The listing builds one solid part. Answer for the finished solid, in the listing's coordinates (mm). Round coordinates to 2 decimals unless told otherwise and drop trailing zeros. Loops run counter-clockwise (first coordinate to the right, second up) from the corner with the lowest first, then second, coordinate; pieces in that order, holes last. Notation, with made-up numbers: (41, 82) - (50, 82) arc R12 ccw to (50, 96) - close; hole circle Ø2 at (-5, -5). An arc over 180 degrees is marked (long way). One line per item, written item: value.
Autodesk Inventor part; units mm, degrees
ref_plane "YZ Plane" through (0, 0, 0) normal (1, 0, 0) x (0, 1, 0)
ref_plane "XZ Plane" through (0, 0, 0) normal (0, 1, 0) x (-1, 0, 0)
ref_plane "XY Plane" through (0, 0, 0) normal (0, 0, 1) x (1, 0, 0)
sketch "Sketch1" plane through (0, 0, 0) normal (0, 0, 1) x (1, 0, 0)
  line L0 (-85.3538, 38.1) -> (162.2962, 38.1)
  line L1 (162.2962, 38.1) -> (162.2962, 12.7)
  line L2 (162.2962, 12.7) -> (-85.3538, 12.7)
  line L3 (-85.3538, 12.7) -> (-85.3538, 38.1)
  line L4 (162.2962, 38.1) -> (115.3062, 38.1)
  line L5 (115.3062, 38.1) -> (115.3062, 0)
  line L6 (115.3062, 0) -> (162.2962, 0)
  line L7 (162.2962, 0) -> (162.2962, 38.1)
  circle A0 centre (-22.5792, -171.9682) radius 173.1686
  line L8 (-85.3538, 12.7) -> (-85.3538, 0)
  line L9 (0, 0) -> (-44.3742, 6.35) construction
  line L10 (-44.3742, 6.35) -> (-85.3538, 0) construction
  spline S0 degree 2 poles (0, 0) (-44.3742, 6.35) (-85.3538, 0) knots 1 1 1 2 2 2
  line L11 (81.5863, -33.6319) -> (69.4058, 12.7)
  line L12 (0, 0) -> (0, 12.7)
  line L13 (0, 0) -> (67.6812, 0)
  line L14 (0, 0) -> (67.6812, 0)
  line L15 (81.5863, -33.6319) -> (29.3756, 0)
  line L16 (0, 0) -> (29.3756, 0)
  line L17 (27.7818, -6.2843) -> (29.3756, 0)
  line L18 (27.7744, -6.2821) -> (21.0977, 0)
  line L19 (7.9763, 0) -> (27.7808, -6.2881)
  line L20 (7.9763, 0) -> (7.5205, -1.4355)
  line L21 (0, 0) -> (7.5205, -1.4355) construction
  spline S1 degree 1 poles (0, 0) (7.5205, -1.4355) knots 1 1 2 2
  line L22 (81.5863, -33.6319) -> (101.3506, -50.0871) construction
  line L23 (101.3506, -50.0871) -> (95.7634, -43.4306) construction
  spline S2 degree 2 poles (81.5863, -33.6319) (101.3506, -50.0871) (95.7634, -43.4306) knots 1 1 1 2 2 2
  line L24 (162.2962, 0) -> (162.2962, -7.7512)
  arc A1 (88.9377, -39.659) -> (162.2962, -7.7512) centre (115.3062, 0) ccw
  arc A2 (162.2962, 7.7512) -> (81.5863, -33.6319) centre (115.3062, 0) ccw
  point P0 (60.3061, -19.9241)
  point P1 (162.2962, 12.7)
  point P2 (115.3062, 12.7)
  point P3 (162.2962, 12.7)
  point P4 (27.497, -6.198)
  point P5 (29.3756, 0)
  point P6 (89.8079, -40.2241)
  dimension "d0" = 247.65
  dimension "d1" = 25.4
  dimension "d4" = 38.1
  dimension "d5" = 46.99
extrude "Extrusion2" add sketch "Sketch1" along normal blind 1.5875 contours L0 A2 L2 L3 | L0 L5 L2 A2 | L2 L12 S0 L8 | L0 A2 L2 L5 | L0 L1 L2 A2 | A2 L13 L12 L2 | L2 L5 L6 L24 A1 A0 L11 | L11 A2 | L2 A2 L7 L6 L5 | L2 L7 A2 | A0 L15 L13 A2 | L13 L20 S1 | A0 L17 L15 | L17 A0 L18 L13 | L13 L18 A0 L19 | L19 A0 L20
fillet "Fillet1" radius 28.575 1 edges at (162.2962, 38.1, 0.7937)
fillet "Fillet2" radius 3.175 1 edges at (-85.3538, 38.1, 0.7937)
fillet "Fillet3" radius 3.175 1 edges at (-85.3538, 0, 0.7937)
sketch "Sketch2" plane through (0, 0, 1.5875) normal (0, 0, 1) x (1, 0, 0)
  circle A0 centre (-77.0322, 20.6187) radius 2.54
  line L0 (-77.0322, 20.6187) -> (-77.0322, 7.9187)
  circle A1 centre (-77.0322, 7.9187) radius 2.54
  line L1 (-77.0322, 20.6187) -> (-13.5322, 20.6187)
  circle A2 centre (-13.5322, 20.6187) radius 2.54
  line L2 (-77.0322, 7.9187) -> (-13.5322, 7.9187)
  circle A3 centre (-13.5322, 7.9187) radius 2.54
  line L3 (-13.5322, 20.6187) -> (-13.5322, 14.2687)
  line L4 (-13.5322, 14.2687) -> (-7.1822, 14.2687)
  circle A4 centre (-7.1822, 14.2687) radius 2.54
  line L5 (-7.1822, 14.2687) -> (5.5178, 14.2687)
  circle A5 centre (5.5178, 14.2687) radius 2.54
  point P0 (0, 0)
  dimension "d15" = 5.08
  dimension "d16" = 12.7
  dimension "d17" = 5.08
  dimension "d18" = 63.5
  dimension "d19" = 5.08
  dimension "d20" = 5.08
  dimension "d21" = 63.5
  dimension "d22" = 6.35
  dimension "d23" = 6.35
  dimension "d24" = 5.08
  dimension "d25" = 12.7
  dimension "d26" = 5.08
properties part number "meers goofy intake sled"
1) Consider L1, parallel to Y at x = -13, z = 0.9; L2, parallel to Y at x = 22.5, z = 0.3; L3, parallel to X at y = -36, z = 0.2. Determine where each line is inside the solid, lowest interval first.
Final values:
L1: 1.6 to 38.1
L2: -4.77 to 38.1
L3: 84.66 to 146.49
2) A cutting plane is placed at A-A on y = -36. Give the vertices of the cut face in (x, z), and give its area (3 significant figures).
Final values:
outline: (84.66, 0) - (146.49, 0) - (146.49, 1.59) - (84.66, 1.59) - close
area: 98.1 mm2
3) A cutting plane is placed at B-B on x = 74. Give the vertices of the cut face in (y, z).
Final values:
outline: (-28.23, 0) - (38.1, 0) - (38.1, 1.59) - (-28.23, 1.59) - close
4) For a pull along Y with two mould halves and no side action, classify faces 1 (the flat face through (64, 5, 1.588)), 2 (the cylindrical face through (135.374, -43.19, 0.783)), 3 (the cylindrical face through (154.148, 29.507, 0.805)) as released by +Y, released by -Y, zero draft, split by the parting line, or undercut.
Final values:
face 1: zero draft
face 2: released by -Y
face 3: released by +Y
5) This flat-tipped pin is pushed along its axis until it touches: pin 1 Ø3 at (x, y) = (-44.5, 15.5) entering from -Z. Where does it stop, or does it pass through?
Final values:
pin 1: z = 0
